Drawing for the job (mm, zero at the part's lowest x, y, z). A direction names the side the tool comes from. Round coordinates to 2 decimals unless told otherwise and drop trailing zeros. Loops run counter-clockwise (first coordinate to the right, second up) from the corner with the lowest first, then second, coordinate; pieces in that order, holes last.
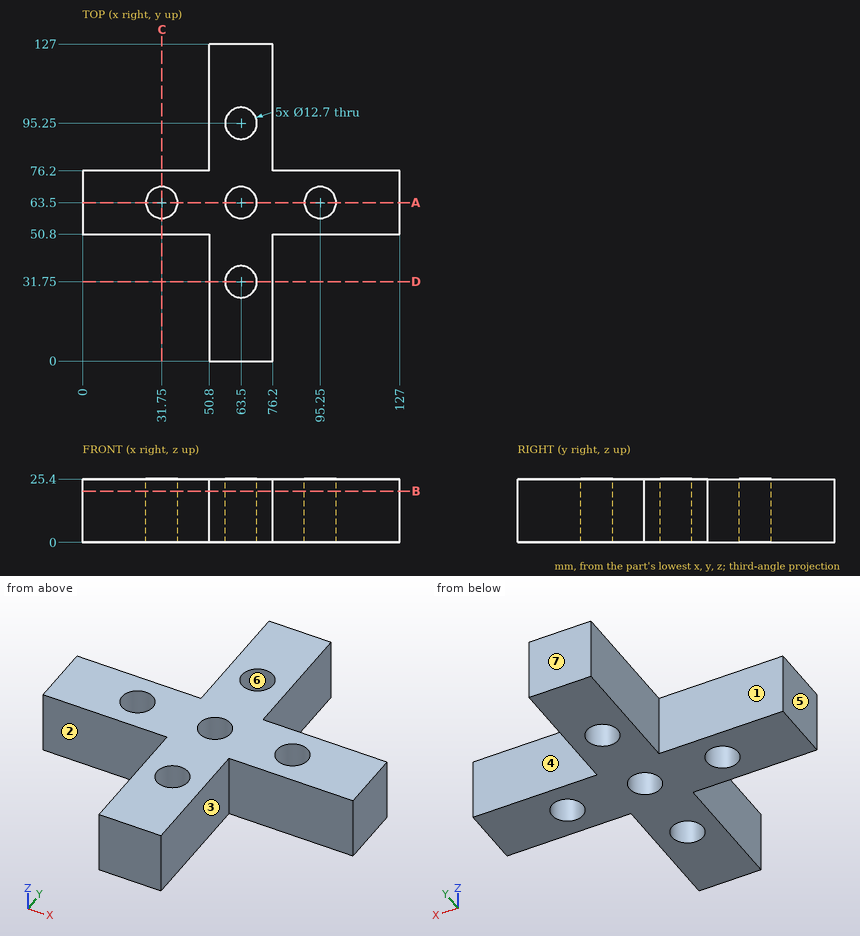
Q1. Slice it at B-B on z = 20.5. Give the cut face in (x, y).
Q2. Pull direction Y, two halves, no side cores. Call the marked faces 5, 6 and 7: pulls with the +Y half, pulls with the -Y half, needs draft (parallel to the pull), parting line crosses it, or undercut.
Q3. Tool access for the marked faces 1, 2, 3 and 4: list every direction of +Z, -Z, +X, -X, +Y, -Y with a clear straight run to the whole face (end or side of a thin tool).
Q4. Probe line 1 (X direction, y = 63.5, z = 5.75); line 2 (X direction, y = 95.25, z = 16.5); line 3 (X direction, y = 8, z = 17). List the from-to ranges inside material, lowest first.
Q5. Slice it at C-C on x = 31.75. Give the cut face in (y, z).
Q6. Slice it at A-A on y = 63.5. Give the cut face in (x, z).
Q7. Flat gauge pins, fed straight in: P1, Ø10, axis at x = 110.5, z = 13.5, coming from the +Y side; P2, Ø16.5, axis at x = 63.5, y = 95.25, coming from the +Z side; P3, Ø4, axis at x = 92.5, z = 11.5, coming from the -Y side; P4, Ø10, axis at x = 31.75, y = 63.5, coming from the -Z side. Where does each tip first touch, or does it go through?
Reply:
1. outline: (0, 50.8) - (50.8, 50.8) - (50.8, 0) - (76.2, 0) - (76.2, 50.8) - (127, 50.8) - (127, 76.2) - (76.2, 76.2) - (76.2, 127) - (50.8, 127) - (50.8, 76.2) - (0, 76.2) - close; hole circle Ø12.7 at (31.75, 63.5); hole circle Ø12.7 at (63.5, 31.75); hole circle Ø12.7 at (63.5, 63.5); hole circle Ø12.7 at (63.5, 95.25); hole circle Ø12.7 at (95.25, 63.5)
2. face 5: needs draft
2. face 6: undercut
2. face 7: pulls with the +Y half
3. face 1: +Z, -Z, -X, +Y
3. face 2: +Z, -Z, -X, -Y
3. face 3: +Z, -Z, +X, -Y
3. face 4: +Z, -Z, +X, +Y
4. line 1: x = 0 to 25.4, 38.1 to 57.15, 69.85 to 88.9, 101.6 to 127
4. line 2: x = 50.8 to 57.15, 69.85 to 76.2
4. line 3: x = 50.8 to 76.2
5. outline: (50.8, 0) - (57.15, 0) - (57.15, 25.4) - (50.8, 25.4) - close; (69.85, 0) - (76.2, 0) - (76.2, 25.4) - (69.85, 25.4) - close
6. outline: (0, 0) - (25.4, 0) - (25.4, 25.4) - (0, 25.4) - close; (38.1, 0) - (57.15, 0) - (57.15, 25.4) - (38.1, 25.4) - close; (69.85, 0) - (88.9, 0) - (88.9, 25.4) - (69.85, 25.4) - close; (101.6, 0) - (127, 0) - (127, 25.4) - (101.6, 25.4) - close
7. P1: stops at y = 76.2
7. P2: stops at z = 25.4
7. P3: stops at y = 50.8
7. P4: passes through
